Autodesk Inventor part; units mm, degrees
ref_plane "YZ Plane" through (0, 0, 0) normal (1, 0, 0) x (0, 1, 0)
ref_plane "XZ Plane" through (0, 0, 0) normal (0, 1, 0) x (-1, 0, 0)
ref_plane "XY Plane" through (0, 0, 0) normal (0, 0, 1) x (1, 0, 0)
sketch "スケッチ1" plane through (0, 0, 0) normal (0, 1, 0) x (-1, 0, 0)
  arc A0 (348.9954, -50.1786) -> (348.3553, -42.2361) centre (348.3204, -46.2359) ccw
  arc A1 (182.359, -65.8653) -> (348.9954, -50.1786) centre (162.2533, 1040.6287) ccw
  arc A2 (135.1603, -65.3257) -> (182.359, -65.8653) centre (167.871, 731.467) ccw
  arc A3 (48.4731, -49.9165) -> (135.1603, -65.3257) centre (148.588, 261.756) ccw
  arc A4 (-1.5687, -25.3375) -> (48.4731, -49.9165) centre (107.173, 132.825) ccw
  arc A5 (-15.7749, -11.5429) -> (-1.5687, -25.3375) centre (31.9, 23.342) ccw
  arc A6 (-8.2474, 11.5993) -> (-15.7749, -11.5429) centre (-3.6695, -2.6851) ccw
  arc A7 (13.0537, 14.3873) -> (-8.2474, 11.5993) centre (10.0641, -45.5382) ccw
  arc A8 (91.047, 0) -> (13.0537, 14.3873) centre (-1.8944, -285.2401) ccw
  arc A9 (91.047, 0) -> (95.8009, -1.5381) centre (462.8125, 1140.9603) ccw
  arc A10 (95.8009, -1.5381) -> (348.3553, -42.2361) centre (355.7675, 807.7316) ccw
  point P0 (0, 0)
extrude "押し出し1" add sketch "スケッチ1" along normal mid plane 4
sketch "スケッチ2" plane through (0, -2, 0) normal (0, -1, 0) x (1, 0, 0)
  line L0 (0, 0) -> (-283.8627, -59.346)
  arc A0 (-348.9954, -50.1786) -> (-182.359, -65.8653) centre (-162.2533, 1040.6287) ccw
  circle A1 centre (-29.3651, -6.1392) radius 6
  circle A2 centre (-239.8151, -50.1371) radius 6
  dimension "d3" = 290
  dimension "d4" = 12
  dimension "d5" = 12
  dimension "d6" = 30
  dimension "d7" = 215
extrude "押し出し2" cut sketch "スケッチ2" against normal through all
properties part number "flap_m"
For this review, take the finished solid that the model builds, in its own axes (mm). Round coordinates to 2 decimals unless told otherwise and drop trailing zeros. Write each loop counter-clockwise with the first axis right and the second up, starting at its lowest first coordinate (ties: lowest second). Pieces come first, ordered by that corner, then holes. Notation, with made-up numbers: M 7.25,0.25 L 29.25,0.25 A31 cw 29.25,28.25 Z; hole C -2,-3.75 d2. An arc over 180 degrees is marked long. Write item = value, one per line. Start each with the question number.
(1) We need section A-A (y = -1.3). Give the boundary of the cut face in (x, z).
(2) Clearance check with flat-ended pins moving along their axes: pin 1 Ø1 at (x, z) = (-190, -23.5) entering from +Y; pin 2 Ø1 at (x, y) = (-23.5, -1.5) entering from -Z; pin 3 Ø1 at (y, z) = (-1, -42) entering from +X. State where each tip first meets the part, or that it passes through.
(3) For line 1 along X through (y, z) = (1.5, -45); line 2 along Z through (x, y) = (-14, 0.75); line 3 along Z through (x, y) = (-271, -1.55), list the stretches that pass through material, from the lowest coordinate up.
(4) The part is to be moulded in two halves that separate along X. For faces 1 (the face through (-34.126, -0.028, -9.79)), 2 (the face through (17.994, -0.028, 1.765)), 3 (the face through (-123, 2, -34)), 4 (the face through (-267.142, -0.028, -61.066)), say which applies: +X half, -X half, draft (parallel to the pull), parting line (faces both ways), or undercut.
(5) We need section B-B (x = -289.5). Give the boundary of the cut face in (y, z), then the cut area to 3 significant figures.
(6) We need section C-C (z = -19.5). Give the boundary of the cut face in (x, y).
Results found:
q1.outline = M -349,-50.18 A1106.67 ccw -182.36,-65.87 A797.54 ccw -135.16,-65.33 A327.36 ccw -48.47,-49.92 A191.94 ccw 1.57,-25.34 A59.07 ccw 15.77,-11.54 A15 ccw 8.25,11.6 A60 ccw -13.05,14.39 A300 ccw -91.05,0 A1211.19 cw -95.8,-1.54 A850 cw -348.36,-42.24 A4 ccw Z; hole C -239.82,-50.14 d12; hole C -29.37,-6.14 d12
q2.pin_1 = through
q2.pin_2 = -40.16
q2.pin_3 = -26.86
q3.line_1 = -352.12 to -242.92, -236.72 to -34.93
q3.line_2 = -34.98 to 14.34
q3.line_3 = -60.69 to -38.03
q4.face_1 = undercut
q4.face_2 = +X half
q4.face_3 = draft
q4.face_4 = -X half
q5.outline = M -2,-58.71 L 2,-58.71 L 2,-39.68 L -2,-39.68 Z
q5.area = 76.1 mm²
q6.outline = M -160.35,-2 L 8.77,-2 L 8.77,2 L -160.35,2 Z
